Geometry: final body of the model. Coordinates: model frame, mm. Give positions to 0.01 mm unless a question says otherwise; leave off trailing zeros. Answer as a JSON object with one key per item and string values.
from build123d import *

# Parameters (mm, degrees)
SKETCH1_W           = 669.8488
SKETCH1_H           = 846.328
BOSS_EXTRUDE1_DEPTH = 19.05
CHAMFER1_SIZE       = 2.54
CHAMFER2_SIZE       = 2.54
CUT_EXTRUDE2_DEPTH  = 670.8488
SKETCH2_R           = 3.175
CUT_EXTRUDE3_DEPTH  = 20.05


with BuildPart() as part:
    # Sketch1 → Boss-Extrude1 (new body)
    with BuildSketch(Plane(origin=(0, 0, 0), x_dir=(1, 0, 0), z_dir=(0, 1, 0))):
        with Locations((334.9244, 423.164)):
            Rectangle(SKETCH1_W, SKETCH1_H)
    extrude(amount=BOSS_EXTRUDE1_DEPTH)

    # Chamfer1
    chamfer1_edges = [part.edges().sort_by_distance(p)[0] for p in [
        (669.8488, 19.05, -423.164),
        (334.9244, 19.05, -846.328),
        (0, 19.05, -423.164),
        (334.9244, 19.05, 0),
    ]]
    chamfer(chamfer1_edges, length=CHAMFER1_SIZE)

    # Chamfer2
    chamfer2_edges = [part.edges().sort_by_distance(p)[0] for p in [
        (334.9244, 0, -846.328),
    ]]
    chamfer(chamfer2_edges, length=CHAMFER2_SIZE)

    # Sketch3 → Cut-Extrude2 (cut, through all)
    with BuildSketch(Plane.ZY):
        Polygon((-580.93356, 5.97535), (-580.93356, 0), (-561.88356, 0), (-561.88356, 5.97535), (-559.21656, 5.97535), (-559.21656, 9.53135), (-583.60056, 9.53135), (-583.60056, 5.97535), align=None)
    extrude(amount=-CUT_EXTRUDE2_DEPTH, mode=Mode.SUBTRACT)

    # Sketch2 → Cut-Extrude3 (cut, through all)
    with BuildSketch(Plane(origin=(0, 19.05, 0), x_dir=(1, 0, 0), z_dir=(0, 1, 0))):
        with Locations((57.15, 568.325)):
            Circle(SKETCH2_R)
        with Locations((57.15, 228.6)):
            Circle(SKETCH2_R)
        with Locations((666.75, 568.325)):
            Circle(SKETCH2_R)
        with Locations((666.75, 228.6)):
            Circle(SKETCH2_R)
    extrude(amount=-CUT_EXTRUDE3_DEPTH, mode=Mode.SUBTRACT)


solid = part.part
1) Pull-direction query (Y, two-part tool) for faces 1 (the flat face through (669.849, 8, -112)), 2 (the flat face through (330, 19.05, -429)), 3 (the flat face through (330, 9.531, -571)), 4 (the flat face through (330, 0, -714)); classes: pulls with the +Y half, pulls with the -Y half, needs draft (parallel to the pull), parting line crosses it, or undercut.
Geometry check:
{"face 1": "needs draft", "face 2": "pulls with the +Y half", "face 3": "undercut", "face 4": "pulls with the -Y half"}
2) Contact query for a flat-ended pin moving along its axis: P1, Ø10, axis at x = 666.75, z = -568.325, coming from the -Y side. Output: stop coordinate, or through.
Geometry check:
{"P1": "stops at y = 9.53"}
3) Line query: line 1 (Z direction, x = 666.75, y = 13.25) (3 decimals); line 2 (Z direction, x = 550.5, y = 6.25); line 3 (X direction, y = 8.75, z = -228.6) (3 decimals). Output: solid intervals per line, ascending. Write a range as from..to.
Geometry check:
{"line 1": "z = -846.328..-571.5, -565.15..-231.775, -225.425..0", "line 2": "z = -846.33..-583.6, -559.22..0", "line 3": "x = 0..53.975, 60.325..663.575"}
